from build123d import *

# Parameters (mm, degrees)
SKETCH1_W               = 19.82
SKETCH1_H               = 39.88
BOSS_EXTRUDE1_DEPTH     = 36.02
SKETCH2_W               = 19.82
SKETCH2_H               = 6.6
BOSS_EXTRUDE2_DEPTH     = 2.54
CUT_EXTRUDE1_DEPTH      = 2.54
SKETCH4_W               = 1
SKETCH4_H               = 6.6
BOSS_EXTRUDE3_DEPTH     = 1.5
CUT_EXTRUDE2_DEPTH      = 10.41
CUT_EXTRUDE2_DEPTH_BACK = 11.41
SKETCH6_W               = 19.82
SKETCH6_H               = 39.88
CUT_EXTRUDE3_DEPTH      = 3.55
SKETCH7_W               = 18.22
SKETCH7_H               = 38.272033082
BOSS_EXTRUDE4_DEPTH     = 0.762
FILLET1_R               = 1.27
FILLET2_R               = 0.762
BOSS_EXTRUDE5_DEPTH     = 2.54
SKETCH9_R               = 6.475
BOSS_EXTRUDE6_DEPTH     = 2.286
SKETCH10_R              = 5.46
BOSS_EXTRUDE7_DEPTH     = 0.762
SKETCH11_R              = 1.75
CUT_EXTRUDE4_DEPTH      = 2.54
SKETCH12_W              = 17.371497452
SKETCH12_H              = 10
SKETCH12_W_2            = 15.851497452
SKETCH12_H_2            = 8.48
BOSS_EXTRUDE8_DEPTH     = 0.254
BOSS_EXTRUDE9_DEPTH     = 2.54
CUT_EXTRUDE5_DEPTH      = 1.524
SKETCH15_R              = 0.5
CUT_EXTRUDE6_DEPTH      = 6
CHAMFER1_SIZE           = 1
FILLET3_R               = 0.5
SKETCH16_W              = 6.35
SKETCH16_H              = 3.686799723
SKETCH16_W_2            = 5.35
SKETCH16_H_2            = 2.686799723
BOSS_EXTRUDE10_DEPTH    = 1.5
FILLET4_R               = 0.5
FILLET5_R               = 1


with BuildPart() as part:
    # Sketch1 → Boss-Extrude1 (new body)
    with BuildSketch(Plane(origin=(0, 0, 0), x_dir=(1, 0, 0), z_dir=(0, 1, 0))):
        Rectangle(SKETCH1_W, SKETCH1_H)
    extrude(amount=BOSS_EXTRUDE1_DEPTH)

    # Sketch2 → Boss-Extrude2 (add)
    with BuildSketch(Plane(origin=(0, 26.67, 0), x_dir=(1, 0, 0), z_dir=(0, 1, 0))):
        with Locations((0, 23.24)):
            Rectangle(SKETCH2_W, SKETCH2_H)
        with Locations((0, -23.24)):
            Rectangle(SKETCH2_W, SKETCH2_H)
    extrude(amount=BOSS_EXTRUDE2_DEPTH)

    # Sketch3 → Cut-Extrude1 (cut)
    with BuildSketch(Plane(origin=(0, 29.21, 0), x_dir=(1, 0, 0), z_dir=(0, 1, 0))):
        with BuildLine():
            Line((-3.56, 26.54), (-6.36, 26.54))
            Line((-6.36, 26.54), (-6.36, 25.544072445))
            ThreePointArc((-6.36, 25.544072445), (-4.96, 21.67), (-3.56, 25.544072445))
            Line((-3.56, 25.544072445), (-3.56, 26.54))
        make_face()
        with BuildLine():
            Line((6.36, 26.54), (3.56, 26.54))
            Line((3.56, 26.54), (3.56, 25.544072445))
            ThreePointArc((3.56, 25.544072445), (4.96, 21.67), (6.36, 25.544072445))
            Line((6.36, 25.544072445), (6.36, 26.54))
        make_face()
    cut_extrude1 = extrude(amount=-CUT_EXTRUDE1_DEPTH, mode=Mode.SUBTRACT)

    # Mirror1: Cut-Extrude1 across plane
    add(cut_extrude1.mirror(Plane.XY), mode=Mode.SUBTRACT)

    # Sketch4 → Boss-Extrude3 (add)
    with BuildSketch(Plane(origin=(0, 29.21, 0), x_dir=(1, 0, 0), z_dir=(0, 1, 0))):
        with Locations((0, 23.24)):
            Rectangle(SKETCH4_W, SKETCH4_H)
        with Locations((0, -23.24)):
            Rectangle(SKETCH4_W, SKETCH4_H)
    extrude(amount=BOSS_EXTRUDE3_DEPTH)

    # Sketch5 → Cut-Extrude2 (cut, two sides)
    with BuildSketch(Plane.ZY.offset(0.5)) as cut_extrude2_sk:
        Polygon((-26.54, 30.71), (-25.54, 30.71), (-26.54, 29.21), align=None)
        Polygon((25.54, 30.71), (26.54, 29.21), (26.54, 30.71), align=None)
    extrude(amount=CUT_EXTRUDE2_DEPTH, mode=Mode.SUBTRACT)
    extrude(cut_extrude2_sk.sketch, amount=-CUT_EXTRUDE2_DEPTH_BACK, mode=Mode.SUBTRACT)

    # Sketch6 → Cut-Extrude3 (cut)
    with BuildSketch(Plane(origin=(0, 36.02, 0), x_dir=(1, 0, 0), z_dir=(0, 1, 0))):
        Rectangle(SKETCH6_W, SKETCH6_H)
    extrude(amount=-CUT_EXTRUDE3_DEPTH, mode=Mode.SUBTRACT)

    # Sketch7 → Boss-Extrude4 (add)
    with BuildSketch(Plane(origin=(0, 32.47, 0), x_dir=(1, 0, 0), z_dir=(0, 1, 0))):
        Rectangle(SKETCH7_W, SKETCH7_H)
    extrude(amount=BOSS_EXTRUDE4_DEPTH)

    # Fillet1
    fillet1_edges = [part.edges().sort_by_distance(p)[0] for p in [
        (-9.91, 13.335, -19.94),
        (9.91, 13.335, -19.94),
        (9.91, 30.84, -19.94),
        (9.91, 30.84, 19.94),
        (-9.91, 30.84, 19.94),
        (-9.91, 30.84, -19.94),
        (9.91, 13.335, 19.94),
        (-9.91, 13.335, 19.94),
    ]]
    fillet(fillet1_edges, radius=FILLET1_R)

    # Fillet2
    fillet2_edges = [part.edges().sort_by_distance(p)[0] for p in [
        (9.11, 32.851, -19.136016541),
        (-9.11, 32.851, -19.136016541),
        (-9.11, 32.851, 19.136016541),
        (9.11, 32.851, 19.136016541),
    ]]
    fillet(fillet2_edges, radius=FILLET2_R)

    # Sketch8 → Boss-Extrude5 (add)
    with BuildSketch(Plane(origin=(0, 33.232, 0), x_dir=(1, 0, 0), z_dir=(0, 1, 0))):
        with BuildLine():
            Line((-8.685748726, -12.786016541), (8.685748726, -12.786016541))
            Line((8.685748726, -12.786016541), (8.685748726, 7.213983459))
            ThreePointArc((8.685748726, 7.213983459), (0, 19.136016541), (-8.685748726, 7.213983459))
            Line((-8.685748726, 7.213983459), (-8.685748726, -12.786016541))
        make_face()
    extrude(amount=BOSS_EXTRUDE5_DEPTH)

    # Sketch9 → Boss-Extrude6 (add)
    with BuildSketch(Plane(origin=(0, 35.772, 0), x_dir=(1, 0, 0), z_dir=(0, 1, 0))):
        with Locations((0, 10.011016541)):
            Circle(SKETCH9_R)
    extrude(amount=BOSS_EXTRUDE6_DEPTH)

    # Sketch10 → Boss-Extrude7 (add)
    with BuildSketch(Plane(origin=(0, 38.058, 0), x_dir=(1, 0, 0), z_dir=(0, 1, 0))):
        with Locations((0, 10.011016541)):
            Circle(SKETCH10_R)
    extrude(amount=BOSS_EXTRUDE7_DEPTH)

    # Sketch11 → Cut-Extrude4 (cut)
    with BuildSketch(Plane(origin=(0, 38.82, 0), x_dir=(1, 0, 0), z_dir=(0, 1, 0))):
        with Locations((0, 10.011016541)):
            Circle(SKETCH11_R)
    extrude(amount=-CUT_EXTRUDE4_DEPTH, mode=Mode.SUBTRACT)

    # Sketch12 → Boss-Extrude8 (add)
    with BuildSketch(Plane(origin=(0, 35.772, 0), x_dir=(1, 0, 0), z_dir=(0, 1, 0))):
        with Locations((0, -7.788983459)):
            Rectangle(SKETCH12_W, SKETCH12_H)
        with Locations((0, -7.788983459)):
            Rectangle(SKETCH12_W_2, SKETCH12_H_2, mode=Mode.SUBTRACT)
    extrude(amount=BOSS_EXTRUDE8_DEPTH)

    # Sketch13 → Boss-Extrude9 (add)
    with BuildSketch(Plane(origin=(0, 33.232, 0), x_dir=(1, 0, 0), z_dir=(0, 1, 0))):
        with BuildLine():
            Line((-4.260837189, -12.79), (4.260837189, -12.79))
            ThreePointArc((4.260837189, -12.79), (0, -14.358983459), (-4.260837189, -12.79))
        make_face()
    extrude(amount=BOSS_EXTRUDE9_DEPTH)

    # Sketch14 → Cut-Extrude5 (cut)
    with BuildSketch(Plane.XZ):
        with BuildLine():
            Line((6.46365167, -19.94), (9.91, -19.94))
            Line((9.91, -19.94), (9.91, -16.211847956))
            ThreePointArc((9.91, -16.211847956), (7.678426739, -17.605953774), (6.46365167, -19.94))
        make_face()
        with BuildLine():
            Line((-9.91, -19.94), (-9.91, -16.211847956))
            ThreePointArc((-9.91, -16.211847956), (-7.678426739, -17.605953774), (-6.46365167, -19.94))
            Line((-6.46365167, -19.94), (-9.91, -19.94))
        make_face()
        with BuildLine():
            Line((-6.46365167, 19.94), (-9.91, 19.94))
            Line((-9.91, 19.94), (-9.91, 16.211847956))
            ThreePointArc((-9.91, 16.211847956), (-7.678426739, 17.605953774), (-6.46365167, 19.94))
        make_face()
        with BuildLine():
            Line((9.91, 19.94), (9.91, 16.211847956))
            ThreePointArc((9.91, 16.211847956), (7.678426739, 17.605953774), (6.46365167, 19.94))
            Line((6.46365167, 19.94), (9.91, 19.94))
        make_face()
    extrude(amount=-CUT_EXTRUDE5_DEPTH, mode=Mode.SUBTRACT)

    # Sketch15 → Cut-Extrude6 (cut)
    with BuildSketch(Plane(origin=(0, 0, 0), x_dir=(-1, 0, 0), z_dir=(0, -1, 0))):
        with Locations((-8.64, 18.67)):
            Circle(SKETCH15_R)
        with Locations((8.64, 18.67)):
            Circle(SKETCH15_R)
        with Locations((8.64, -18.67)):
            Circle(SKETCH15_R)
        with Locations((-8.64, -18.67)):
            Circle(SKETCH15_R)
    extrude(amount=-CUT_EXTRUDE6_DEPTH, mode=Mode.SUBTRACT)

    # Chamfer1
    chamfer1_edges = [part.edges().sort_by_distance(p)[0] for p in [
        (0, 0, 19.94),
        (-9.91, 0, 0),
        (0, 0, -19.94),
        (9.91, 0, 0),
    ]]
    chamfer(chamfer1_edges, length=CHAMFER1_SIZE)

    # Fillet3
    fillet3_edges = [part.edges().sort_by_distance(p)[0] for p in [
        (7.678426739, 1.524, 17.605953774),
        (-7.678426739, 1.524, 17.605953774),
        (-7.678426739, 1.524, -17.605953774),
        (7.678426739, 1.524, -17.605953774),
    ]]
    fillet(fillet3_edges, radius=FILLET3_R)

    # Sketch16 → Boss-Extrude10 (add)
    with BuildSketch(Plane(origin=(0, 0, -19.94), x_dir=(-1, 0, 0), z_dir=(0, 0, -1))):
        with Locations((0, 2.843399862)):
            Rectangle(SKETCH16_W, SKETCH16_H)
        with Locations((0, 2.843399862)):
            Rectangle(SKETCH16_W_2, SKETCH16_H_2, mode=Mode.SUBTRACT)
    extrude(amount=BOSS_EXTRUDE10_DEPTH)

    # Fillet4
    fillet4_edges = [part.edges().sort_by_distance(p)[0] for p in [
        (3.175, 4.686799723, -20.69),
        (3.175, 1, -20.69),
        (-3.175, 1, -20.69),
        (-3.175, 4.686799723, -20.69),
    ]]
    fillet(fillet4_edges, radius=FILLET4_R)

    # Fillet5
    fillet5_edges = [part.edges().sort_by_distance(p)[0] for p in [
        (-9.91, 27.94, -26.54),
        (9.91, 27.94, -26.54),
        (-9.91, 27.94, 26.54),
        (9.91, 27.94, 26.54),
    ]]
    fillet(fillet5_edges, radius=FILLET5_R)


solid = part.part
Work out the finished part from the listing and answer in its coordinate system (mm). A direction names the side the tool comes from. Give positions to 0.01 mm unless a question says otherwise; leave off trailing zeros. Loops run counter-clockwise (first coordinate to the right, second up) from the corner with the lowest first, then second, coordinate; pieces in that order, holes last. Notation, with made-up numbers: M 68,41.25 L 86,41.25 A34 ccw 86,74.25 Z; hole C 63.25,52.25 d6. An arc over 180 degrees is marked long. Use CSV: the item, a comma, the result in double quotes.
1) Find section A-A on z = 23.86. Write down the section's boundary in (x, y), plus the area to 3 significant figures.
Answer:
outline,"M -9.91,26.67 L -7.15,26.67 L -7.15,29.21 L -9.91,29.21 Z; M -2.77,26.67 L 2.77,26.67 L 2.77,29.21 L 0.5,29.21 L 0.5,30.71 L -0.5,30.71 L -0.5,29.21 L -2.77,29.21 Z; M 7.15,26.67 L 9.91,26.67 L 9.91,29.21 L 7.15,29.21 Z"
area,"29.6 mm^2"
2) Consider L1, parallel to X at y = 27.65, z = 23.86; L2, parallel to X at y = 3.95, z = 18.67; L3, parallel to Z at x = -8.64, y = 4.4. Determine where each line is inside the solid, lowest interval first.
Answer:
L1,"-9.91 to -7.15, -2.77 to 2.77, 7.15 to 9.91"
L2,"-9.91 to -9.14, -8.14 to 8.14, 9.14 to 9.91"
L3,"-19.94 to -19.17, -18.17 to 18.17, 19.17 to 19.94"
3) Given P1, Ø6, axis at x = -4, y = 20, coming from the -Z side; P2, Ø10, axis at x = -1.5, z = -19, coming from the -Y side; P3, Ø4, axis at x = -3.5, y = 5, coming from the +Z side; P4, Ø1.6, axis at y = 3, z = -21, coming from the -X side (3 decimals), each flat-ended and moving along its own axis, determine where each tip first touches the part or whether it passes through.
Answer:
P1,"z = -19.94"
P2,"y = 0"
P3,"z = 19.94"
P4,"x = -3.175"
4) Find section B-B on y = 21. Write down the section's boundary in (x, z).
Answer:
outline,"M -9.91,-18.67 A1.27 ccw -8.64,-19.94 L 8.64,-19.94 A1.27 ccw 9.91,-18.67 L 9.91,18.67 A1.27 ccw 8.64,19.94 L -8.64,19.94 A1.27 ccw -9.91,18.67 Z"
5) Determine the mould class of faces 1 (the cylindrical face through (-5.04, 27.96, -21.67)), 2 (the cylindrical face through (-0.84, 36.9, -16.43)), 3 (the flat face through (-9, 1.524, -18)) for opening direction X: released by +X, released by -X, zero draft, split by the parting line, or undercut.
Answer:
face 1,"undercut"
face 2,"split by the parting line"
face 3,"zero draft"
6) Which of the six approach directions +Z, -Z, +X, -X, +Y, -Y give full straight-line access (tool end or side, diameter ignored) to faces 4 (the flat face through (6.2, 29.21, 21.7)), 5 (the flat face through (0, 3, -19.94)), 6 (the flat face through (-7, 33.232, -17)), 7 (the flat face through (-0.5, 30, 23)), 8 (the cylindrical face through (7.7, 0.5, -17.58))?
Answer:
face 4,"+Z, +X, +Y"
face 5,"-Z"
face 6,"-Z, -X, +Y"
face 7,"+Z, -X, +Y"
face 8,"-Z, +X, -Y"
7) Find section C-C on z = 7.5. Write down the section's boundary in (x, y).
Answer:
outline,"M -9.91,1 L -8.91,0 L 8.91,0 L 9.91,1 L 9.91,32.47 L 9.11,32.47 L 9.11,33.23 L 8.69,33.23 L 8.69,36.03 L 7.93,36.03 L 7.93,35.77 L -7.93,35.77 L -7.93,36.03 L -8.69,36.03 L -8.69,33.23 L -9.11,33.23 L -9.11,32.47 L -9.91,32.47 Z"
